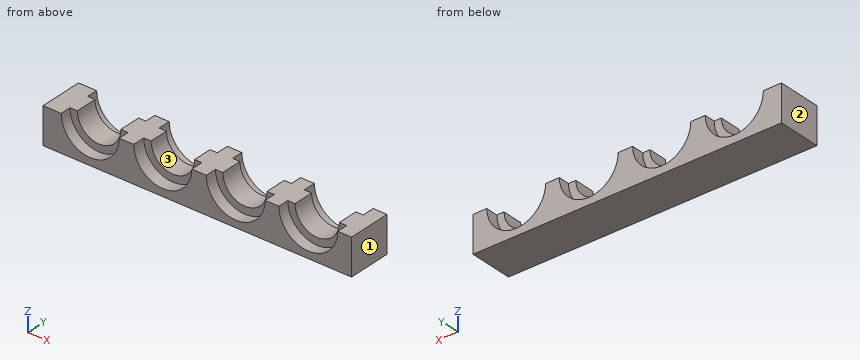
```python
from build123d import *

# Parameters (mm, degrees)
F1_W     = 85
F1_H     = 12
F2_DEPTH = 10


with BuildPart() as f2:
    # F1 (on Top) → F2 (new body)
    with BuildSketch(Plane.XY):
        with Locations((42.5, 6)):
            Rectangle(F1_W, F1_H)
    extrude(amount=F2_DEPTH)

    # F3 (on offset) → F4 (revolve, cut)
    with BuildSketch(Plane.XY.offset(10)):
        Polygon((5, 3), (5, 0), (13, 0), (13, 12), (5, 12), (5, 9), (7, 9), (7, 3), align=None)
    revolve(axis=Axis((13, 6, 10), (0, 1, 0)), mode=Mode.SUBTRACT)

    # F5 (on offset) → F6 (revolve, cut)
    with BuildSketch(Plane.XY.offset(10)):
        Polygon((25, 3.4), (25, 0), (33, 0), (33, 12), (25, 12), (25, 8.6), (27, 8.6), (27, 3.4), align=None)
    revolve(axis=Axis((33, 6, 10), (0, 1, 0)), mode=Mode.SUBTRACT)

    # F7 (on offset) → F8 (revolve, cut)
    with BuildSketch(Plane.XY.offset(10)):
        Polygon((45, 3.1), (45, 0), (53.1, 0), (53.1, 12), (45, 12), (45, 8.9), (47, 8.9), (47, 3.1), align=None)
    revolve(axis=Axis((53.1, 6, 10), (0, 1, 0)), mode=Mode.SUBTRACT)

    # F9 (on offset) → F10 (revolve, cut)
    with BuildSketch(Plane.XY.offset(10)):
        Polygon((65, 3), (65, 0), (73.1, 0), (73.1, 12), (65, 12), (65, 8.6), (67, 8.6), (67, 3), align=None)
    revolve(axis=Axis((73.1, 6, 10), (0, 1, 0)), mode=Mode.SUBTRACT)


solid = f2.part
```
CAD build for the part. Positions are in the model's coordinates, mm. Face numbers are marked on the shaded views. Coordinates: 2 decimals unless noted, no trailing zeros. Loops run counter-clockwise (first coordinate to the right, second up) from the corner with the lowest first, then second, coordinate; pieces in that order, holes last. Notation, with made-up numbers: (-30.5, -39) - (21.5, -39) arc R12 ccw to (21.5, -34) - close; hole circle Ø3 at (68.25, 0.25). An arc over 180 degrees is marked (long way). Use CSV: the item, a comma, the result in double quotes. Start each with the question number.
Q1. Cut at C-C, the plane z = 7.25. State how many separate pieces and enclosed holes the cut face has, then the cut area to 3 significant figures.
Q2. Cut at B-B, the plane y = 5. List the corners of the cut face in (x, z), then the cut area to 3 significant figures.
Q3. Cut at D-D, the plane x = 73.1. List the corners of the cut face in (y, z).
Q4. Drop flat-ended pins along their axis: P1, Ø2.5, axis at x = 12.5, z = 6, coming from the -Y side; P2, Ø4, axis at x = 72, z = 5, coming from the -Y side; P3, Ø4, axis at x = 56, z = 6.5, coming from the -Y side; P4, Ø2.5, axis at x = 29.5, z = 5.5, coming from the -Y side. Give the stop position or say it passes through.
Q5. Cut at A-A, the plane x = 13. List the corners of the cut face in (y, z), then the cut area to 3 significant figures.
Q6. Probe probe 1 along X at (y, z) = (9.75, 3); probe 2 along X at (y, z) = (7, 4.5); probe 3 along Y at (x, z) = (18, 5.5). List the from-to ranges inside material, lowest first. Write a range as from..to.
Q7. Two-plate mould, pull along X, no slides. Class the marked faces 1, 2 and 3: +X half, -X half, draft (parallel to the pull), parting line (faces both ways), or undercut.
Here are the results:
1,separate pieces,"5"
1,enclosed holes,"0"
1,area,"392 mm2"
2,outline,"(0, 0) - (85, 0) - (85, 10) - (79.2, 10) arc R6.1 cw to (67, 10) - (59.2, 10) arc R6.1 cw to (47, 10) - (39, 10) arc R6 cw to (27, 10) - (19, 10) arc R6 cw to (7, 10) - (0, 10) - close"
2,area,"620 mm2"
3,outline,"(0, 0) - (12, 0) - (12, 1.9) - (8.6, 1.9) - (8.6, 3.9) - (3, 3.9) - (3, 1.9) - (0, 1.9) - close"
4,P1,"through"
4,P2,"y = 3"
4,P3,"y = 3.1"
4,P4,"y = 3.4"
5,outline,"(0, 0) - (12, 0) - (12, 2) - (9, 2) - (9, 4) - (3, 4) - (3, 2) - (0, 2) - close"
5,area,"36.0 mm2"
6,probe 1,"0..9.13, 16.87..29.13, 36.87..49.02, 57.18..69.02, 77.18..85"
6,probe 2,"0..10.6, 15.4..30.6, 35.4..50.46, 55.74..70.46, 75.74..85"
6,probe 3,"3..9"
7,face 1,"+X half"
7,face 2,"-X half"
7,face 3,"undercut"
